Read the model definition and answer for the solid it produces. Units are mm, in the model's axes. Give positions to 0.01 mm unless a question says otherwise; leave off trailing zeros. Loops run counter-clockwise (first coordinate to the right, second up) from the corner with the lowest first, then second, coordinate; pieces in that order, holes last. Notation, with made-up numbers: (46.25, 79) - (59.25, 79) arc R5 cw to (59.25, 85) - close; hole circle Ø6 at (34, 57.5). An arc over 180 degrees is marked (long way). Write item = value, one per line.
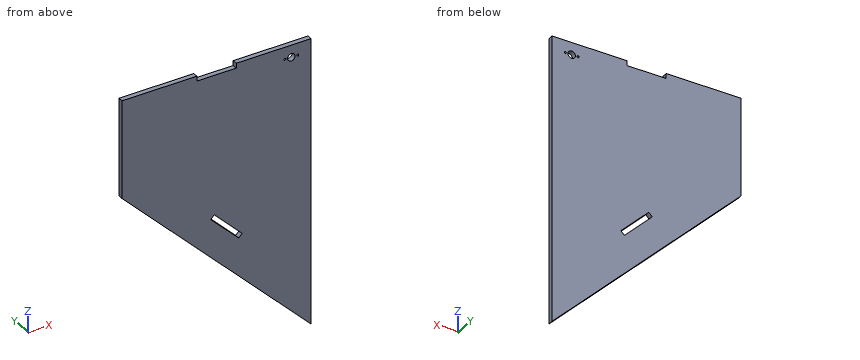
```python
from build123d import *

# Parameters (mm, degrees)
BOSS_EXTRUDE1_DEPTH = 3.175
SKETCH2_R           = 2.38125
SKETCH2_R_2         = 0.635
SKETCH2_W           = 25.4
SKETCH2_H           = 3.175
CUT_EXTRUDE1_DEPTH  = 3.175


with BuildPart() as part:
    # Sketch1 → Boss-Extrude1 (new body)
    with BuildSketch(Plane(origin=(0, 0, 0), x_dir=(1, 0, 0), z_dir=(0, 1, 0))):
        Polygon((0, 63.5), (121.871664787, 185.371664787), (121.871664787, 121.549227353), (121.871664787, 0), (63.5, 0), (31.75, 0), (0, 0), align=None)
    extrude(amount=BOSS_EXTRUDE1_DEPTH)

    # Sketch2 → Cut-Extrude1 (cut)
    with BuildSketch(Plane(origin=(0, 3.175, 0), x_dir=(1, 0, 0), z_dir=(0, 1, 0))):
        with Locations(Location((109.171664787, 7.8994, 0), (0, 0, 270))):
            Circle(SKETCH2_R)
        with Locations(Location((105.044164787, 7.8994, 0), (0, 0, 270))):
            Circle(SKETCH2_R_2)
        with Locations(Location((113.299164787, 7.8994, 0), (0, 0, 270))):
            Circle(SKETCH2_R_2)
        Polygon((57.240266841, 96.06229437), (59.485330871, 93.81723034), (77.445843113, 111.777742582), (75.200779083, 114.022806612), align=None)
        with Locations((60.96, 1.5875)):
            Rectangle(SKETCH2_W, SKETCH2_H)
    extrude(amount=-CUT_EXTRUDE1_DEPTH, mode=Mode.SUBTRACT)


solid = part.part
```
1) A cutting plane is placed at B-B on z = -126. Determine the outline of the cut face in (x, y) (3 decimals).
Output:
outline = (62.5, 0) - (121.872, 0) - (121.872, 3.175) - (62.5, 3.175) - close
2) A cutting plane is placed at C-C on x = 100.5. Determine the outline of the cut face in (y, z) (3 decimals), then the cut area to 3 significant figures.
Output:
outline = (0, -164) - (3.175, -164) - (3.175, 0) - (0, 0) - close
area = 521 mm²
3) Each of these flat-tipped pins is pushed along its axis until it touches: P1, Ø1.5, axis at y = 1.5, z = -117, coming from the -X side; P2, Ø6, axis at x = 66.5, z = -24.5, coming from the -Y side. Where does it stop, or does it pass through?
Output:
P1 = 52.75
P2 = 0
4) Find the intervals of material crossed by probe 1 along Z at (x, y) = (57.5, 1.2) (3 decimals); probe 2 along Z at (x, y) = (109.5, 1); probe 3 along X at (y, z) = (0.6, -141), in increasing order.
Output:
probe_1 = -121 to -96.322, -95.803 to -3.175
probe_2 = -173 to -10.26, -5.54 to 0
probe_3 = 77.5 to 121.87
5) A cutting plane is placed at A-A on y = 1.6. Determine the outline of the cut face in (x, z) (1 decimal), then the cut area to 3 significant figures.
Output:
outline = (0, -63.5) - (121.9, -185.4) - (121.9, 0) - (73.7, 0) - (73.7, -3.2) - (48.3, -3.2) - (48.3, 0) - (0, 0) - close; hole (57.2, -96.1) - (75.2, -114) - (77.4, -111.8) - (59.5, -93.8) - close; hole circle Ø1.3 at (105, -7.9); hole circle Ø4.8 at (109.2, -7.9); hole circle Ø1.3 at (113.3, -7.9)
area = 15,000 mm²
